Study the drawing (mm; zero at the part's minimum x, y, z) and answer. Coordinates: 2 decimals unless noted, no trailing zeros. Write each loop counter-clockwise with the first axis right and the second up, starting at its lowest first coordinate (ties: lowest second). Pieces come first, ordered by that corner, then holes. Notation, with made-up numbers: (87, 27) -> (126, 27) arc R26 ccw to (126, 62) -> close; hole circle Ø3 at (-9, 2). An arc over 180 degrees is marked (long way). Answer in a Markdown table with one row per item. Add a question column.
Item 1: Section D-D on x = 8 is taken. Write down the section's boundary in (y, z), then the cut area to 3 significant figures.
Item 2: Straight lines are drawn through the part: line 1 (X direction, y = 7.5, z = 21); line 2 (Y direction, x = 1, z = 30.5); line 3 (Y direction, x = 6.5, z = 33). For each, find the intervals that lie inside material, in ascending order. Write a range as from..to.
Item 3: Section B-B on z = 36 is taken. Write down the section's boundary in (x, y).
Item 4: Section A-A on x = 6 is taken. Write down the section's boundary in (y, z), then the cut area to 3 significant figures.
Item 5: Given pin 1 Ø1.5 at (x, y) = (6.5, 11) entering from +Z; pin 2 Ø4 at (x, z) = (2.5, 16) entering from +Y; pin 3 Ø2 at (y, z) = (9.5, 2) entering from +X, each flat-ended and moving along its own axis, determine where each tip first touches the part or whether it passes through.
Item 6: Section C-C on y = 3 is taken. Write down the section's boundary in (x, z).
Item 7: For a pull along X with two mould halves and no side action, classify the marked faces 1, 2 and 3 as +X half, -X half, draft (parallel to the pull), parting line (faces both ways), or undercut.
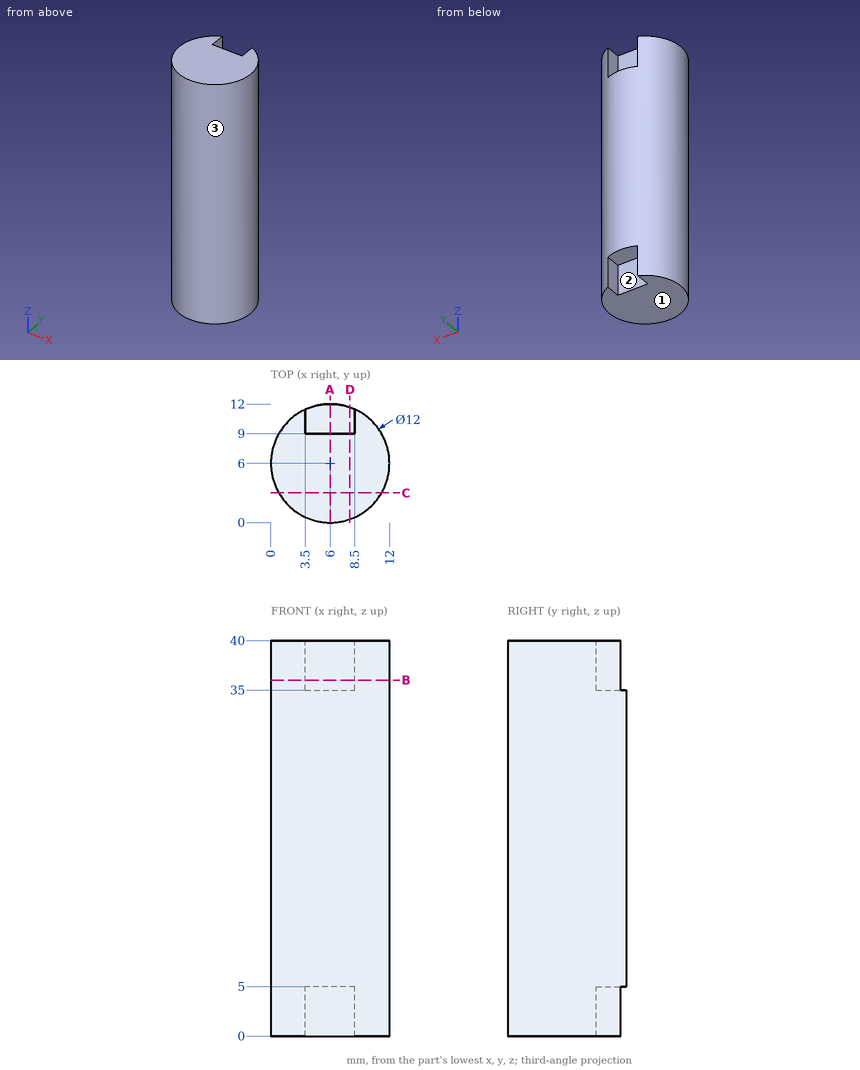
Results below:
| question | item | result |
|---|---|---|
| 1 | outline | (0.34, 0) -> (9, 0) -> (9, 5) -> (11.66, 5) -> (11.66, 35) -> (9, 35) -> (9, 40) -> (0.34, 40) -> close |
| 1 | area | 426 mm2 |
| 2 | line 1 | x = 0.19..11.81 |
| 2 | line 2 | y = 2.68..9.32 |
| 2 | line 3 | y = 0.02..11.98 |
| 3 | outline | (3.5, 9) -> (3.5, 11.45) arc R6 ccw (long way) to (8.5, 11.45) -> (8.5, 9) -> close |
| 4 | outline | (0, 0) -> (9, 0) -> (9, 5) -> (12, 5) -> (12, 35) -> (9, 35) -> (9, 40) -> (0, 40) -> close |
| 4 | area | 450 mm2 |
| 5 | pin 1 | stops at z = 35 |
| 5 | pin 2 | stops at y = 11.81 |
| 5 | pin 3 | stops at x = 11.45 |
| 6 | outline | (0.8, 0) -> (11.2, 0) -> (11.2, 40) -> (0.8, 40) -> close |
| 7 | face 1 | draft |
| 7 | face 2 | undercut |
| 7 | face 3 | parting line |
